Verification items for the finished model (mm, model axes). Face numbers are marked on the shaded views. A direction names the side the tool comes from. Coordinates: 2 decimals unless noted, no trailing zeros. Order: outer loops, then holes, each group sorted by start corner. A loop starts at its lowest first (then second) coordinate and runs counter-clockwise, first axis right, second up. Notation, with made-up numbers: M -10,25.5 L 30,25.5 A17 cw 30,52.5 Z; hole C 16,47 d2. An arc over 180 degrees is marked long. Return JSON: item names as keys, results as strings.
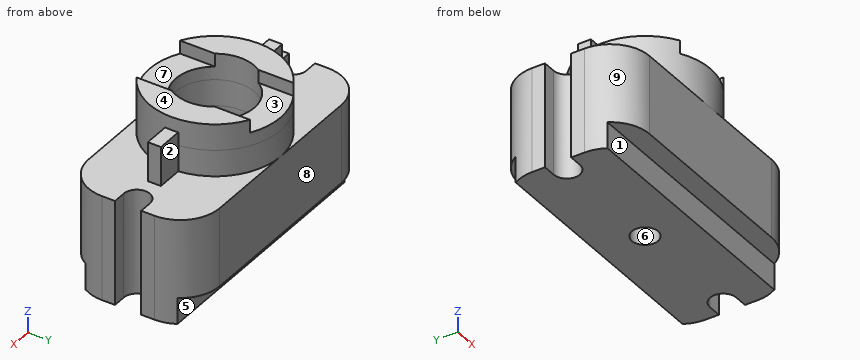
```python
from build123d import *

# Parameters (mm, degrees)
SKETCH1_W           = 200
SKETCH1_H           = 100
BOSS_EXTRUDE1_DEPTH = 100
CUT_EXTRUDE2_DEPTH  = 100
CUT_EXTRUDE3_DEPTH  = 100
SKETCH4_W           = 20
SKETCH4_H           = 15
CUT_EXTRUDE8_DEPTH  = 275
SKETCH8_R           = 10
CUT_EXTRUDE9_DEPTH  = 275
SKETCH9_R           = 30
SKETCH9_R_2         = 10
CUT_EXTRUDE10_DEPTH = 50
SKETCH10_R          = 50
SKETCH10_R_2        = 30
BOSS_EXTRUDE2_DEPTH = 20
CUT_EXTRUDE12_DEPTH = 10
SKETCH12_W          = 20
SKETCH12_H          = 10
BOSS_EXTRUDE3_DEPTH = 10
SKETCH13_W          = 20
SKETCH13_H          = 10
BOSS_EXTRUDE4_DEPTH = 10
CUT_EXTRUDE13_DEPTH = 20
SKETCH15_R          = 50
SKETCH15_R_2        = 30
BOSS_EXTRUDE5_DEPTH = 20
SKETCH16_W          = 20
SKETCH16_H          = 10
BOSS_EXTRUDE6_DEPTH = 30


with BuildPart() as part:
    # Sketch1 → Boss-Extrude1 (new body)
    with BuildSketch(Plane.XY):
        with Locations((100, 50)):
            Rectangle(SKETCH1_W, SKETCH1_H)
    extrude(amount=BOSS_EXTRUDE1_DEPTH)

    # Sketch2 → Cut-Extrude2 (cut)
    with BuildSketch(Plane.XY.offset(100)):
        with BuildLine():
            Line((30, 100), (0, 100))
            Line((0, 100), (0, 70))
            ThreePointArc((0, 70), (8.786796564, 91.213203436), (30, 100))
        make_face()
        with BuildLine():
            Line((200, 100), (170, 100))
            ThreePointArc((170, 100), (191.213203436, 91.213203436), (200, 70))
            Line((200, 70), (200, 100))
        make_face()
        with BuildLine():
            Line((200, 0), (200, 30))
            ThreePointArc((200, 30), (191.213203436, 8.786796564), (170, 0))
            Line((170, 0), (200, 0))
        make_face()
        with BuildLine():
            ThreePointArc((30, 0), (8.786796564, 8.786796564), (0, 30))
            Line((0, 30), (0, 0))
            Line((0, 0), (30, 0))
        make_face()
    extrude(amount=-CUT_EXTRUDE2_DEPTH, mode=Mode.SUBTRACT)

    # Sketch3 → Cut-Extrude3 (cut)
    with BuildSketch(Plane.XY.offset(100)):
        with BuildLine():
            Line((10, 60), (0, 60))
            Line((0, 60), (0, 40))
            Line((0, 40), (10, 40))
            ThreePointArc((10, 40), (20, 50), (10, 60))
        make_face()
        with BuildLine():
            Line((190, 60), (200, 60))
            Line((200, 60), (200, 40))
            Line((200, 40), (190, 40))
            ThreePointArc((190, 40), (180, 50), (190, 60))
        make_face()
    extrude(amount=-CUT_EXTRUDE3_DEPTH, mode=Mode.SUBTRACT)

    # Sketch4 → Cut-Extrude8 (cut)
    with BuildSketch(Plane(origin=(0, 0, 0), x_dir=(0, 0, -1), z_dir=(1, 0, 0))):
        with Locations((-10, 92.5)):
            Rectangle(SKETCH4_W, SKETCH4_H)
        with Locations((-10, 7.5)):
            Rectangle(SKETCH4_W, SKETCH4_H)
    extrude(amount=CUT_EXTRUDE8_DEPTH, mode=Mode.SUBTRACT)

    # Sketch8 → Cut-Extrude9 (cut)
    with BuildSketch(Plane.XY.offset(100)):
        with Locations((100, 50)):
            Circle(SKETCH8_R)
    extrude(amount=-CUT_EXTRUDE9_DEPTH, mode=Mode.SUBTRACT)

    # Sketch9 → Cut-Extrude10 (cut)
    with BuildSketch(Plane.XY.offset(100)):
        with Locations((100, 50)):
            Circle(SKETCH9_R)
        with Locations((100, 50)):
            Circle(SKETCH9_R_2, mode=Mode.SUBTRACT)
    extrude(amount=-CUT_EXTRUDE10_DEPTH, mode=Mode.SUBTRACT)

    # Sketch10 → Boss-Extrude2 (add)
    with BuildSketch(Plane.XY.offset(100)):
        with Locations((100, 50)):
            Circle(SKETCH10_R)
        with Locations((100, 50)):
            Circle(SKETCH10_R_2, mode=Mode.SUBTRACT)
    extrude(amount=BOSS_EXTRUDE2_DEPTH)

    # Sketch11 → Cut-Extrude12 (cut)
    with BuildSketch(Plane.XY.offset(120)):
        with BuildLine():
            ThreePointArc((125, 93.301270189), (100, 100), (75, 93.301270189))
            Line((75, 93.301270189), (75, 66.583123952))
            ThreePointArc((75, 66.583123952), (100, 80), (125, 66.583123952))
            Line((125, 66.583123952), (125, 93.301270189))
        make_face()
        with BuildLine():
            Line((75, 33.416876048), (75, 6.698729811))
            ThreePointArc((75, 6.698729811), (100, 0), (125, 6.698729811))
            Line((125, 6.698729811), (125, 33.416876048))
            ThreePointArc((125, 33.416876048), (100, 20), (75, 33.416876048))
        make_face()
    extrude(amount=-CUT_EXTRUDE12_DEPTH, mode=Mode.SUBTRACT)

    # Sketch12 → Boss-Extrude3 (add)
    with BuildSketch(Plane.XY.offset(100)):
        with Locations((40.250628145, 50)):
            Rectangle(SKETCH12_W, SKETCH12_H)
    extrude(amount=BOSS_EXTRUDE3_DEPTH)

    # Sketch13 → Boss-Extrude4 (add)
    with BuildSketch(Plane.XY.offset(100)):
        with Locations((159.749371855, 50)):
            Rectangle(SKETCH13_W, SKETCH13_H)
    extrude(amount=BOSS_EXTRUDE4_DEPTH)

    # Sketch14 → Cut-Extrude13 (cut)
    with BuildSketch(Plane.XY.offset(100)):
        with BuildLine():
            ThreePointArc((200, 30), (191.213203436, 8.786796564), (170, 0))
            Line((170, 0), (170, 100))
            ThreePointArc((170, 100), (191.213203436, 91.213203436), (200, 70))
            Line((200, 70), (200, 60))
            Line((200, 60), (190, 60))
            ThreePointArc((190, 60), (180, 50), (190, 40))
            Line((190, 40), (200, 40))
            Line((200, 40), (200, 30))
        make_face()
        with BuildLine():
            Line((170, 100), (100, 100))
            ThreePointArc((100, 100), (66.458980338, 87.080992435), (50.250628145, 55))
            Line((50.250628145, 55), (30.250628145, 55))
            Line((30.250628145, 55), (30.250628145, 45))
            Line((30.250628145, 45), (50.250628145, 45))
            ThreePointArc((50.250628145, 45), (66.458980338, 12.919007565), (100, 0))
            Line((100, 0), (170, 0))
            Line((170, 0), (170, 100))
        make_face()
        with BuildLine():
            Line((30, 100), (30, 0))
            Line((30, 0), (100, 0))
            ThreePointArc((100, 0), (66.458980338, 12.919007565), (50.250628145, 45))
            Line((50.250628145, 45), (30.250628145, 45))
            Line((30.250628145, 45), (30.250628145, 55))
            Line((30.250628145, 55), (50.250628145, 55))
            ThreePointArc((50.250628145, 55), (66.458980338, 87.080992435), (100, 100))
            Line((100, 100), (30, 100))
        make_face()
        with BuildLine():
            Line((30, 100), (30, 0))
            ThreePointArc((30, 0), (8.786796564, 8.786796564), (0, 30))
            Line((0, 30), (0, 40))
            Line((0, 40), (10, 40))
            ThreePointArc((10, 40), (20, 50), (10, 60))
            Line((10, 60), (0, 60))
            Line((0, 60), (0, 70))
            ThreePointArc((0, 70), (8.786796564, 91.213203436), (30, 100))
        make_face()
    extrude(amount=-CUT_EXTRUDE13_DEPTH, mode=Mode.SUBTRACT)

    # Sketch15 → Boss-Extrude5 (add)
    with BuildSketch(Plane(origin=(0, 0, 100), x_dir=(-1, 0, 0), z_dir=(0, 0, -1))):
        with Locations((-100, 50)):
            Circle(SKETCH15_R)
        with Locations((-100, 50)):
            Circle(SKETCH15_R_2, mode=Mode.SUBTRACT)
    extrude(amount=BOSS_EXTRUDE5_DEPTH)

    # Sketch16 → Boss-Extrude6 (add)
    with BuildSketch(Plane.XY.offset(110)):
        with Locations((40.250628145, 50)):
            Rectangle(SKETCH16_W, SKETCH16_H)
        with Locations((159.749371855, 50)):
            Rectangle(SKETCH16_W, SKETCH16_H)
    extrude(amount=-BOSS_EXTRUDE6_DEPTH)


solid = part.part
```
Q1. Tool access check on the marked faces 1, 2, 3, 4 and 5. Record the directions out of +Z, -Z, +X, -X, +Y, -Y that give a thin tool (end or side, any length) a straight path to the whole face; none if there is none.
Values:
{"face 1": "-Z, +X, -X, -Y", "face 2": "+Z, +X, +Y", "face 3": "+Z, +Y, -Y", "face 4": "+Z, +X, -X, +Y, -Y", "face 5": "-Z, +X, -X, +Y"}
Q2. Cross-section at A-A, the plane y = 50. Record the boundary of the cut face in (x, z).
Values:
{"outline": "M 20,0 L 90,0 L 90,50 L 70,50 L 70,120 L 50,120 L 50,110 L 30.25,110 L 30.25,80 L 20,80 Z; M 110,0 L 180,0 L 180,80 L 169.75,80 L 169.75,110 L 150,110 L 150,120 L 130,120 L 130,50 L 110,50 Z"}
Q3. Material ranges on line 1 along X through (y, z) = (50, 85); line 2 along Y through (x, z) = (100, 35); line 3 along Y through (x, z) = (100, 105.5), recorded low to high.
Values:
{"line 1": "30.25 to 70, 130 to 169.75", "line 2": "0 to 40, 60 to 100", "line 3": "0 to 20, 80 to 100"}
Q4. Draft check along X on the marked faces 6, 7, 8 and 9. Enter one of: pulls with the +X half, pulls with the -X half, needs draft (parallel to the pull), parting line crosses it, or undercut.
Values:
{"face 6": "undercut", "face 7": "undercut", "face 8": "needs draft", "face 9": "pulls with the -X half"}
Q5. Cross-section at D-D, the plane y = 89. Record the boundary of the cut face in (x, z), and give its area (3 significant figures).
Values:
{"outline": "M 6.78,20 L 193.22,20 L 193.22,80 L 131.29,80 L 131.29,120 L 125,120 L 125,110 L 75,110 L 75,120 L 68.71,120 L 68.71,80 L 6.78,80 Z", "area": "13,200 mm^2"}
Q6. Go/stop test with flat-tipped pins: pin 1 (5 mm diameter, centred on y = 15, z = 116, fed in from -X); pin 2 (6 mm diameter, centred on y = 29, z = 73.5, fed in from -X); pin 3 (3 mm diameter, centred on y = 48.5, z = 92.5, fed in from +X); pin 4 (11 mm diameter, centred on x = 38, y = 49.5, fed in from +Z). Record where each tip stops, or that it passes through.
Values:
{"pin 1": "x = 62", "pin 2": "x = 0", "pin 3": "x = 169.75", "pin 4": "z = 110"}
Q7. Cross-section at C-C, the plane x = 83. Record the boundary of the cut face in (y, z), and give its area (3 significant figures).
Values:
{"outline": "M 0,20 L 15,20 L 15,0 L 85,0 L 85,20 L 100,20 L 100,80 L 97.02,80 L 97.02,110 L 74.72,110 L 74.72,50 L 25.28,50 L 25.28,110 L 2.98,110 L 2.98,80 L 0,80 Z", "area": "7,260 mm^2"}
Q8. Cross-section at B-B, the plane z = 26. Record the boundary of the cut face in (x, y).
Values:
{"outline": "M 0,30 A30 ccw 30,0 L 170,0 A30 ccw 200,30 L 200,40 L 190,40 A10 cw 190,60 L 200,60 L 200,70 A30 ccw 170,100 L 30,100 A30 ccw 0,70 L 0,60 L 10,60 A10 cw 10,40 L 0,40 Z; hole C 100,50 d20"}
